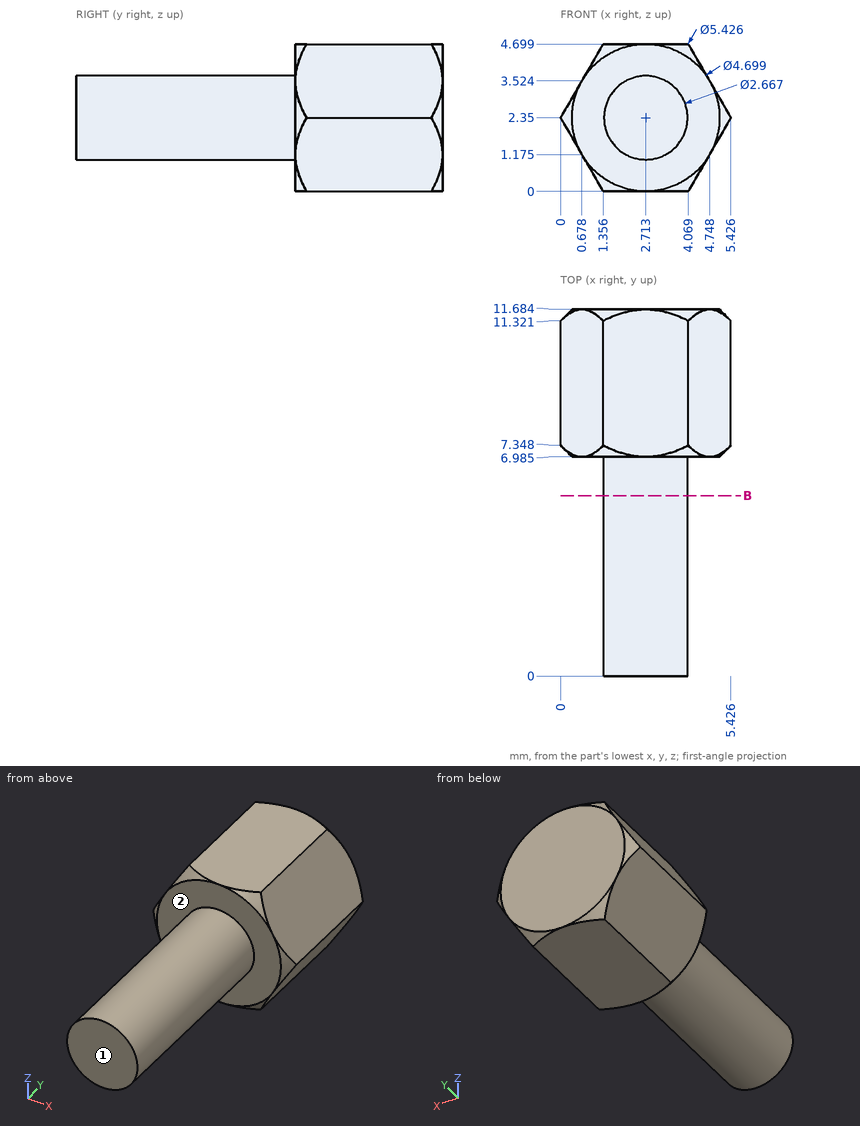
Job drawing, mm, ordinate dimensions from the low corner. One solid piece. A direction names the side the tool comes from. Round coordinates to 2 decimals unless told otherwise and drop trailing zeros. Write each loop counter-clockwise with the first axis right and the second up, starting at its lowest first coordinate (ties: lowest second). Pieces come first, ordered by that corner, then holes. Notation, with made-up numbers: (5.25, 5.25) -> (56.25, 5.25) arc R7 cw to (56.25, 13.25) -> close; hole circle Ø3 at (-29.75, 0.5). An arc over 180 degrees is marked (long way). Answer as CSV lines item,"result".
1. Tool access for the marked faces 1 and 2: list every direction of +Z, -Z, +X, -X, +Y, -Y with a clear straight run to the whole face (end or side of a thin tool).
Resolved:
face 1,"+Z, -Z, +X, -X, -Y"
face 2,"-Y"
2. Slice it at B-B, the plane y = 5.75. List the corners of the cut face in (x, z).
Resolved:
outline,"circle Ø2.67 at (2.71, 2.35)"
3. Drill centre lines: line 1 (Z direction, x = 2.75, y = 4.5); line 2 (Y direction, x = 4.85, z = 1.8) (1 decimal); line 3 (X direction, y = 9.5, z = 2.5) (1 decimal). Where is each one in solid material? Low to high.
Resolved:
line 1,"1.02 to 3.68"
line 2,"7 to 11.7"
line 3,"0.1 to 5.3"
4. Pin check, flat tips, straight feed: pin 1 Ø2 at (y, z) = (5.5, 3.5) entering from -X; pin 2 Ø1.5 at (x, y) = (4.5, 6.5) entering from +Z. Stop position of each tip, or through.
Resolved:
pin 1,"x = 1.39"
pin 2,"z = 4.43"
